The model under review builds one solid part; all positions refer to its coordinate system, in mm. Face numbers are marked on the shaded views. A direction names the side the tool comes from. Give positions to 0.01 mm unless a question says otherwise; leave off trailing zeros. Write each loop counter-clockwise with the first axis right and the second up, starting at its lowest first coordinate (ties: lowest second). Pieces come first, ordered by that corner, then holes. Notation, with made-up numbers: (69, 4) - (110, 4) arc R25 cw to (110, 38) - close; hole circle Ø3 at (66, 48.25). An arc over 180 degrees is marked (long way). Write item = value, one per line.
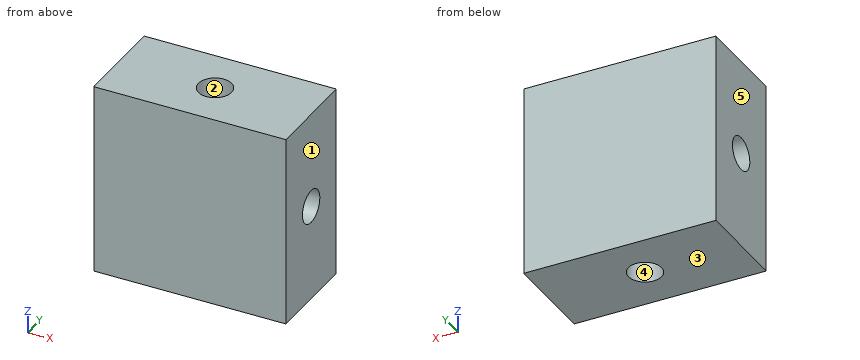
```python
from build123d import *

# Parameters (mm, degrees)
SKETCH1_W           = 20
SKETCH1_H           = 20
BOSS_EXTRUDE1_DEPTH = 5
CIRPATTERN1_COUNT   = 4


with BuildPart() as part:
    # Sketch1 → Boss-Extrude1 (new, symmetric)
    with BuildSketch(Plane(origin=(0, 0, 0), x_dir=(1, 0, 0), z_dir=(0, 1, 0))):
        Rectangle(SKETCH1_W, SKETCH1_H)
    extrude(amount=BOSS_EXTRUDE1_DEPTH, both=True)

    # Sketch3 → #8-32 Tapped Hole1 (revolve, cut)
    with BuildSketch(Plane(origin=(10, 0, 0), x_dir=(0, 0, -1), z_dir=(0, 1, 0))):
        Polygon((0, 0), (0, 7.387806461), (1.7272, 6.35), (1.7272, 0), align=None)
    f_8_32_tapped_hole1 = revolve(axis=Axis((16.35, 0, 0), (-1, 0, 0)), mode=Mode.SUBTRACT)

    # CirPattern1: #8-32 Tapped Hole1 ×4 about axis
    cirpattern1_axis = Axis((0, 0, 0), (0, 1, 0))
    for i in range(1, CIRPATTERN1_COUNT):
        add(f_8_32_tapped_hole1.rotate(cirpattern1_axis, i * 360 / CIRPATTERN1_COUNT), mode=Mode.SUBTRACT)


solid = part.part
```
1. Machinability: for the marked faces 1 and 2, which of the approach directions +Z, -Z, +X, -X, +Y, -Y give a long, thin tool a straight path to every point of the face, cutting with its end or side? Answer none if there is none.
Findings below:
face_1 = +Z, -Z, +X, +Y, -Y
face_2 = +Z
2. Take a section at A-A on x = -5.5. Give the boundary of the cut face in (y, z).
Findings below:
outline = (-5, -10) - (5, -10) - (5, 10) - (-5, 10) - close; hole circle Ø3.45 at (0, 0)
3. Insertion check: P1, Ø3, axis at y = 0, z = 0, coming from the +X side; P2, Ø2, axis at x = 0, y = 0, coming from the -Z side. Each pin has a flat end and moves straight along its axis. Give the tip position at first contact, or say it passes through.
Findings below:
P1 = 3.51
P2 = -3.21
4. Draft analysis for pull direction X (two halves, no side actions). For the marked faces 3, 4 and 5, state which applies: +X half, -X half, draft (parallel to the pull), parting line (faces both ways), or undercut.
Findings below:
face_3 = draft
face_4 = undercut
face_5 = -X half
5. Take a section at B-B on z = 5.25. Give the boundary of the cut face in (x, y).
Findings below:
outline = (-10, -5) - (10, -5) - (10, 5) - (-10, 5) - close; hole circle Ø3.45 at (0, 0)
6. For line 1 (Y direction, x = 0, z = 6.25); line 2 (Z direction, x = 8.5, y = 0), list the stretches that pass through material, from the lowest coordinate up. Write a range as from..to.
Findings below:
line_1 = -5..-1.73, 1.73..5
line_2 = -10..-1.73, 1.73..10
